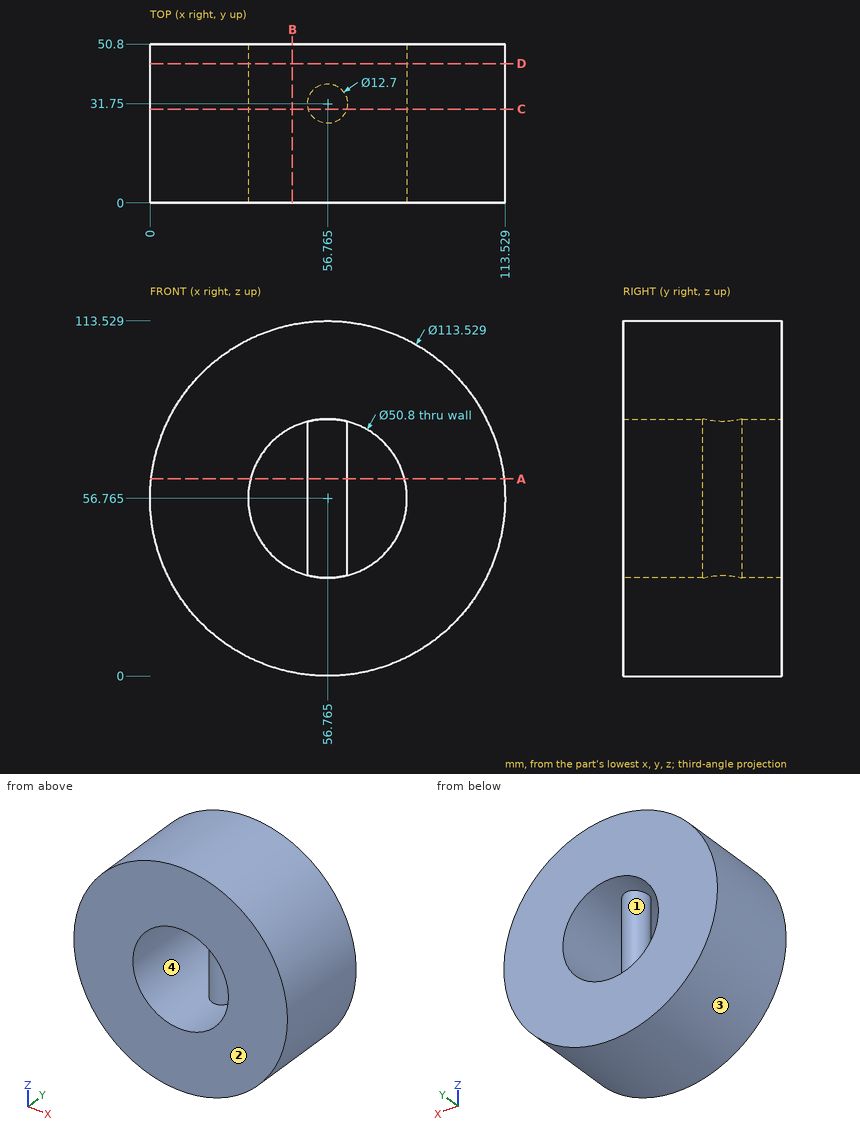
Input: dimensioned drawing with shaded views. Units: mm. Origin: part minimum x, y, z. Coordinates: 2 decimals unless noted, no trailing zeros. Loops run counter-clockwise (first coordinate to the right, second up) from the corner with the lowest first, then second, coordinate; pieces in that order, holes last. Notation, with made-up numbers: M 89.5,2.5 L 144.5,2.5 A14 ccw 144.5,15.5 Z; hole C -24.75,12 d2. An arc over 180 degrees is marked long. Put each result on its own line as item: value.
(1) Cut plane C-C on y = 30. Return the cut outline in (x, z) (1 decimal), then the cut area to 3 significant figures.
Answer sheet:
outline: C 56.8,56.8 d113.5; hole M 50.7,32.1 L 50.7,81.4 A25.4 ccw Z; hole M 62.9,32.1 A25.4 ccw 62.9,81.4 Z
area: 8,710 mm^2
(2) Cut plane B-B on x = 45.5. Return the cut outline in (y, z).
Answer sheet:
outline: M 0,1.13 L 50.8,1.13 L 50.8,34 L 0,34 Z; M 0,79.53 L 50.8,79.53 L 50.8,112.4 L 0,112.4 Z
(3) Material intervals for probe 1 along X at (y, z) = (11, 36) (1 decimal); probe 2 along X at (y, z) = (13, 52.5) (1 decimal); probe 3 along X at (y, z) = (31.5, 34) (1 decimal), sorted ascending.
Answer sheet:
probe 1: x = 3.9 to 42.1, 71.4 to 109.6
probe 2: x = 0.2 to 31.7, 81.8 to 113.4
probe 3: x = 4.8 to 45.5, 50.4 to 63.1, 68 to 108.8
(4) Draft query along X for the marked faces 1, 2, 3 and 4. Return one class per face: pulls with the +X half, pulls with the -X half, needs draft (parallel to the pull), parting line crosses it, or undercut.
Answer sheet:
face 1: undercut
face 2: needs draft
face 3: parting line crosses it
face 4: undercut
(5) Cut plane D-D on y = 44.5. Return the cut outline in (x, z) (1 decimal), then the cut area to 3 significant figures.
Answer sheet:
outline: C 56.8,56.8 d113.5; hole C 56.8,56.8 d50.8
area: 8,100 mm^2
(6) Cut plane A-A on z = 63. State how many separate pieces and enclosed holes the cut face has, then the cut area to 3 significant figures.
Answer sheet:
separate pieces: 3
enclosed holes: 0
area: 3,360 mm^2
(7) First-contact query: pin 1 (1 mm diameter, centred on y = 38.5, z = 71, fed in from -X); pin 2 (6 mm diameter, centred on x = 63.5, y = 27.5, fed in from +Z); pin 3 (12 mm diameter, centred on x = 45.5, y = 41, fed in from +Z) (1 decimal). Flat tips, straight axial feed; report the tip coordinate or a pass-through.
Answer sheet:
pin 1: stops at x = 1.69
pin 2: stops at z = 113.41
pin 3: stops at z = 113.3
